Design review of the part built by this model. Coordinates are the model's own, in mm. Face numbers are marked on the shaded views. A direction names the side the tool comes from. Coordinates: 2 decimals unless noted, no trailing zeros. Loops run counter-clockwise (first coordinate to the right, second up) from the corner with the lowest first, then second, coordinate; pieces in that order, holes last. Notation, with made-up numbers: (80, 61) - (135, 61) arc R21 cw to (135, 91) - close; hole circle Ø5 at (-34, 66). An arc over 180 degrees is marked (long way). One line per question, with ' | ' between items.
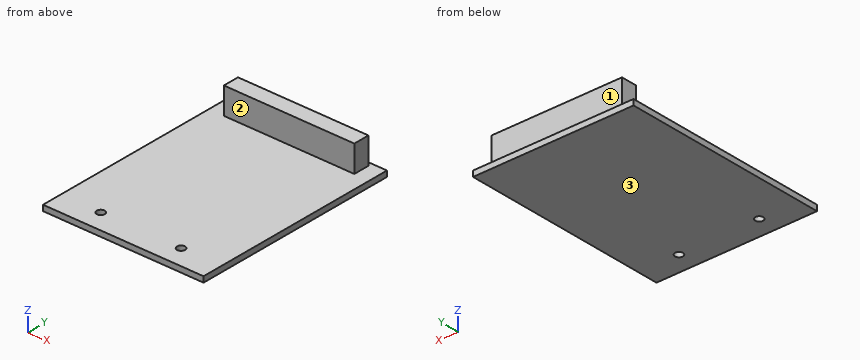
from build123d import *

# Parameters (mm, degrees)
SKETCH1_W           = 50.8
SKETCH1_H           = 66.04
BOSS_EXTRUDE1_DEPTH = 1.778
SKETCH2_W           = 41.275
SKETCH2_H           = 5.08
BOSS_EXTRUDE2_DEPTH = 8.382
SKETCH3_R           = 1.27
CUT_EXTRUDE1_DEPTH  = 1.778


with BuildPart() as part:
    # Sketch1 → Boss-Extrude1 (new body)
    with BuildSketch(Plane.XY):
        with Locations((25.4, 33.02)):
            Rectangle(SKETCH1_W, SKETCH1_H)
    extrude(amount=BOSS_EXTRUDE1_DEPTH)

    # Sketch2 → Boss-Extrude2 (add)
    with BuildSketch(Plane.XY.offset(1.778)):
        with Locations((25.4, 62.23)):
            Rectangle(SKETCH2_W, SKETCH2_H)
    extrude(amount=BOSS_EXTRUDE2_DEPTH)

    # Sketch3 → Cut-Extrude1 (cut)
    with BuildSketch(Plane.XY.offset(1.778)):
        with Locations((12.7, 6.35)):
            Circle(SKETCH3_R)
        with Locations((38.1, 6.35)):
            Circle(SKETCH3_R)
    extrude(amount=-CUT_EXTRUDE1_DEPTH, mode=Mode.SUBTRACT)


solid = part.part
Q1. Take a section at A-A (x = 12.7). Give the boundary of the cut face in (y, z).
Returned:
outline: (0, 0) - (5.08, 0) - (5.08, 1.78) - (0, 1.78) - close; (7.62, 0) - (66.04, 0) - (66.04, 1.78) - (64.77, 1.78) - (64.77, 10.16) - (59.69, 10.16) - (59.69, 1.78) - (7.62, 1.78) - close
Q2. Take a section at B-B (y = 6.35). Give the boundary of the cut face in (x, z), plus the area to 3 significant figures.
Returned:
outline: (0, 0) - (11.43, 0) - (11.43, 1.78) - (0, 1.78) - close; (13.97, 0) - (36.83, 0) - (36.83, 1.78) - (13.97, 1.78) - close; (39.37, 0) - (50.8, 0) - (50.8, 1.78) - (39.37, 1.78) - close | area: 81.3 mm²
Q3. Take a section at C-C (z = 7.25). Give the boundary of the cut face in (x, y).
Returned:
outline: (4.76, 59.69) - (46.04, 59.69) - (46.04, 64.77) - (4.76, 64.77) - close
Q4. Tool access review of the marked faces 1, 2 and 3: name each direction out of +Z, -Z, +X, -X, +Y, -Y from which nothing blocks a thin tool from reaching the whole face with its end or side.
Returned:
face 1: +Z, +X, -X, +Y | face 2: +Z, +X, -X, -Y | face 3: -Z, +X, -X, +Y, -Y
Q5. To check wall thickness, follow line 1 along Y through (x, z) = (12.7, 1.3); line 2 along Z through (x, y) = (45, 13); line 3 along Y through (x, z) = (34.5, 9.75). State the ranges of each line that lie inside material, in increasing order.
Returned:
line 1: y = 0 to 5.08, 7.62 to 66.04 | line 2: z = 0 to 1.78 | line 3: y = 59.69 to 64.77
Q6. For pin 1 (1.5 mm diameter, centred on y = 63, z = 7, fed in from +X); pin 2 (4 mm diameter, centred on x = 34.5, z = 7, fed in from -Y); pin 3 (2.5 mm diameter, centred on y = 62, z = 5, fed in from -X), all flat-tipped, find the tip position at first contact; note any pin that passes through.
Returned:
pin 1: stops at x = 46.04 | pin 2: stops at y = 59.69 | pin 3: stops at x = 4.76
Q7. Take a section at D-D (x = 25). Give the boundary of the cut face in (y, z).
Returned:
outline: (0, 0) - (66.04, 0) - (66.04, 1.78) - (64.77, 1.78) - (64.77, 10.16) - (59.69, 10.16) - (59.69, 1.78) - (0, 1.78) - close
